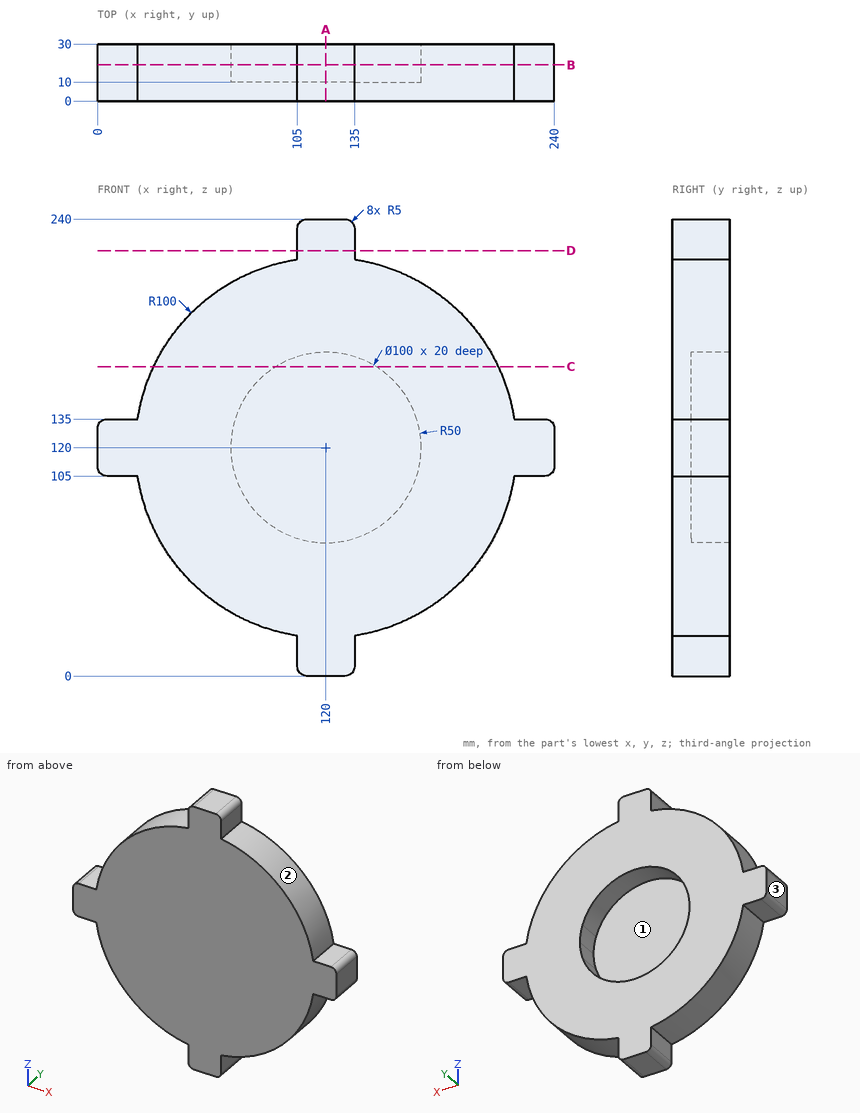
Answer from the drawing. Dimensions are ordinates in mm from the lowest x, y and z of the part. Round coordinates to 2 decimals unless told otherwise and drop trailing zeros. Loops run counter-clockwise (first coordinate to the right, second up) from the corner with the lowest first, then second, coordinate; pieces in that order, holes last.
1) For a pull along Z with two mould halves and no side action, classify the marked faces 1, 2 and 3 as released by +Z, released by -Z, zero draft, split by the parting line, or undercut.
Outcome:
face 1: undercut
face 2: released by +Z
face 3: zero draft
2) A cutting plane is placed at C-C on z = 162.5. Determine the outline of the cut face in (x, y).
Outcome:
outline: (29.48, 0) - (210.52, 0) - (210.52, 30) - (146.34, 30) - (146.34, 10) - (93.66, 10) - (93.66, 30) - (29.48, 30) - close
3) A cutting plane is placed at D-D on z = 223.5. Determine the outline of the cut face in (x, y).
Outcome:
outline: (105, 0) - (135, 0) - (135, 30) - (105, 30) - close
4) Given P1, Ø5, axis at x = 227.5, y = 16.5, coming from the -Z side; P2, Ø13, axis at y = 8, z = 229.5, coming from the -X side; P3, Ø1, axis at x = 161, z = 209.5, coming from the -Y side; P4, Ø1, axis at y = 26.5, z = 95, coming from the -X side, each flat-ended and moving along its own axis, determine where each tip first touches the part or whether it passes through.
Outcome:
P1: stops at z = 105
P2: stops at x = 105
P3: stops at y = 0
P4: stops at x = 23.05
5) Consider line 1 (Z direction, x = 120, y = 18.75); line 2 (X direction, y = 16, z = 117). Determine where each line is inside the solid, lowest interval first.
Outcome:
line 1: z = 0 to 70, 170 to 240
line 2: x = 0 to 70.09, 169.91 to 240
6) A cutting plane is placed at B-B on y = 19. Determine the outline of the cut face in (x, z).
Outcome:
outline: (0, 110) arc R5 ccw to (5, 105) - (21.13, 105) arc R100 ccw to (105, 21.13) - (105, 5) arc R5 ccw to (110, 0) - (130, 0) arc R5 ccw to (135, 5) - (135, 21.13) arc R100 ccw to (218.87, 105) - (235, 105) arc R5 ccw to (240, 110) - (240, 130) arc R5 ccw to (235, 135) - (218.87, 135) arc R100 ccw to (135, 218.87) - (135, 235) arc R5 ccw to (130, 240) - (110, 240) arc R5 ccw to (105, 235) - (105, 218.87) arc R100 ccw to (21.13, 135) - (5, 135) arc R5 ccw to (0, 130) - close; hole circle Ø100 at (120, 120)
7) A cutting plane is placed at A-A on x = 120. Determine the outline of the cut face in (y, z), plus the area to 3 significant figures.
Outcome:
outline: (0, 0) - (30, 0) - (30, 70) - (10, 70) - (10, 170) - (30, 170) - (30, 240) - (0, 240) - close
area: 5,200 mm2
